Part model, mm, in its own coordinate system. A direction names the side the tool comes from. Coordinates: 2 decimals unless noted, no trailing zeros. Loops run counter-clockwise (first coordinate to the right, second up) from the corner with the lowest first, then second, coordinate; pieces in that order, holes last. Notation, with made-up numbers: (74.5, 26) - (83.5, 26) arc R25 ccw to (83.5, 46) - close; hole circle Ø5 at (84.25, 77.5). An arc over 180 degrees is marked (long way). Use a Markdown table: item, result. Add a question column.
1. Drop flat-ended pins along their axis: pin 1 (1.5 mm diameter, centred on x = -5, y = 12.5, fed in from -Z); pin 2 (5 mm diameter, centred on x = 3.5, z = 13, fed in from -Y); pin 3 (5 mm diameter, centred on x = -13, y = -12.5, fed in from +Z). Give the stop position or say it passes through.
2. Band-saw the part on C-C, the plane y = -11. Give the cut face in (x, z).
3. Band-saw the part on B-B, the plane x = 0. Give the cut face in (y, z).
4. 3-axis set-ups, long thin cutter, end or side, ignore diameter. For faces 1 (the cylindrical face through (0, 19, 4)), 2 (the flat face through (-4, 17.75, 6)), 3 (the flat face through (-10, -19, 13)), 4 (the flat face through (4, 19, 14)): which of +Z, -Z, +X, -X, +Y, -Y reach the whole face in a straight line?
5. Band-saw the part on A-A, the plane z = 15. Give the cut face in (x, y).
6. Wall check: probe 1 along X at (y, z) = (7.5, 16); probe 2 along Y at (x, z) = (-7, 4.75); probe 3 along Z at (x, y) = (9.5, 15). Give the ranges that are in metal, low to high. Write a range as [from, to].
7. Pull direction X, two halves, no side cores. Call faces 5 (the flat face through (0, -19, 7)), 6 (the flat face through (-4.2, 19.25, 9.4)), 7 (the flat face through (-17.75, 0, 9)): pulls with the +X half, pulls with the -X half, needs draft (parallel to the pull), parting line crosses it, or undercut.
8. Band-saw the part on D-D, the plane z = 6.5. Give the cut face in (x, y).
from build123d import *

# Parameters (mm, degrees)
ESQUISSE1_W             = 35.5
ESQUISSE1_H             = 38.5
BOSS_EXTRU_1_DEPTH      = 19
ESQUISSE3_W             = 32.5
ESQUISSE3_H             = 35.5
ENL_V_MAT_EXTRU_1_DEPTH = 16
ESQUISSE4_R             = 4
ENL_V_MAT_EXTRU_2_DEPTH = 5
ESQUISSE5_W             = 20
ESQUISSE5_H             = 12
ENL_V_MAT_EXTRU_3_DEPTH = 5


with BuildPart() as part:
    # Esquisse1 → Boss.-Extru.1 (new body)
    with BuildSketch(Plane.XY):
        Rectangle(ESQUISSE1_W, ESQUISSE1_H)
    extrude(amount=BOSS_EXTRU_1_DEPTH)

    # Esquisse3 → Enlèv. mat.-Extru.1 (cut)
    with BuildSketch(Plane.XY.offset(19)):
        Rectangle(ESQUISSE3_W, ESQUISSE3_H)
    extrude(amount=-ENL_V_MAT_EXTRU_1_DEPTH, mode=Mode.SUBTRACT)

    # Esquisse4 → Enlèv. mat.-Extru.2 (cut)
    with BuildSketch(Plane(origin=(0, 19.25, 0), x_dir=(1, 0, 0), z_dir=(0, 1, 0))):
        with BuildLine():
            ThreePointArc((4, -8), (0, -12), (-4, -8))
            Line((-4, -8), (-4, -19))
            Line((-4, -19), (4, -19))
            Line((4, -19), (4, -8))
        make_face()
        with Locations((0, -8)):
            Circle(ESQUISSE4_R)
    extrude(amount=-ENL_V_MAT_EXTRU_2_DEPTH, mode=Mode.SUBTRACT)

    # Esquisse5 → Enlèv. mat.-Extru.3 (cut)
    with BuildSketch(Plane.XZ.offset(19.25)):
        with Locations((0, 13)):
            Rectangle(ESQUISSE5_W, ESQUISSE5_H)
    extrude(amount=-ENL_V_MAT_EXTRU_3_DEPTH, mode=Mode.SUBTRACT)


solid = part.part
Geometry check:
| question | item | result |
|---|---|---|
| 1 | pin 1 | stops at z = 0 |
| 1 | pin 2 | stops at y = 17.75 |
| 1 | pin 3 | stops at z = 3 |
| 2 | outline | (-17.75, 0) - (17.75, 0) - (17.75, 19) - (16.25, 19) - (16.25, 3) - (-16.25, 3) - (-16.25, 19) - (-17.75, 19) - close |
| 3 | outline | (-19.25, 0) - (19.25, 0) - (19.25, 4) - (17.75, 4) - (17.75, 3) - (-17.75, 3) - (-17.75, 7) - (-19.25, 7) - close |
| 4 | face 1 | +Z, +Y |
| 4 | face 2 | +Z |
| 4 | face 3 | +Z, -Y |
| 4 | face 4 | +Z, +Y, -Y |
| 5 | outline | (-17.75, -19.25) - (-10, -19.25) - (-10, -17.75) - (-16.25, -17.75) - (-16.25, 17.75) - (-4, 17.75) - (-4, 19.25) - (-17.75, 19.25) - close; (4, 17.75) - (16.25, 17.75) - (16.25, -17.75) - (10, -17.75) - (10, -19.25) - (17.75, -19.25) - (17.75, 19.25) - (4, 19.25) - close |
| 6 | probe 1 | x = [-17.75, -16.25], [16.25, 17.75] |
| 6 | probe 2 | y = [-19.25, -17.75], [17.75, 19.25] |
| 6 | probe 3 | z = [0, 3] |
| 7 | face 5 | undercut |
| 7 | face 6 | needs draft |
| 7 | face 7 | pulls with the -X half |
| 8 | outline | (-17.75, -19.25) - (17.75, -19.25) - (17.75, 19.25) - (3.71, 19.25) - (3.71, 17.75) - (16.25, 17.75) - (16.25, -17.75) - (-16.25, -17.75) - (-16.25, 17.75) - (-3.71, 17.75) - (-3.71, 19.25) - (-17.75, 19.25) - close |
